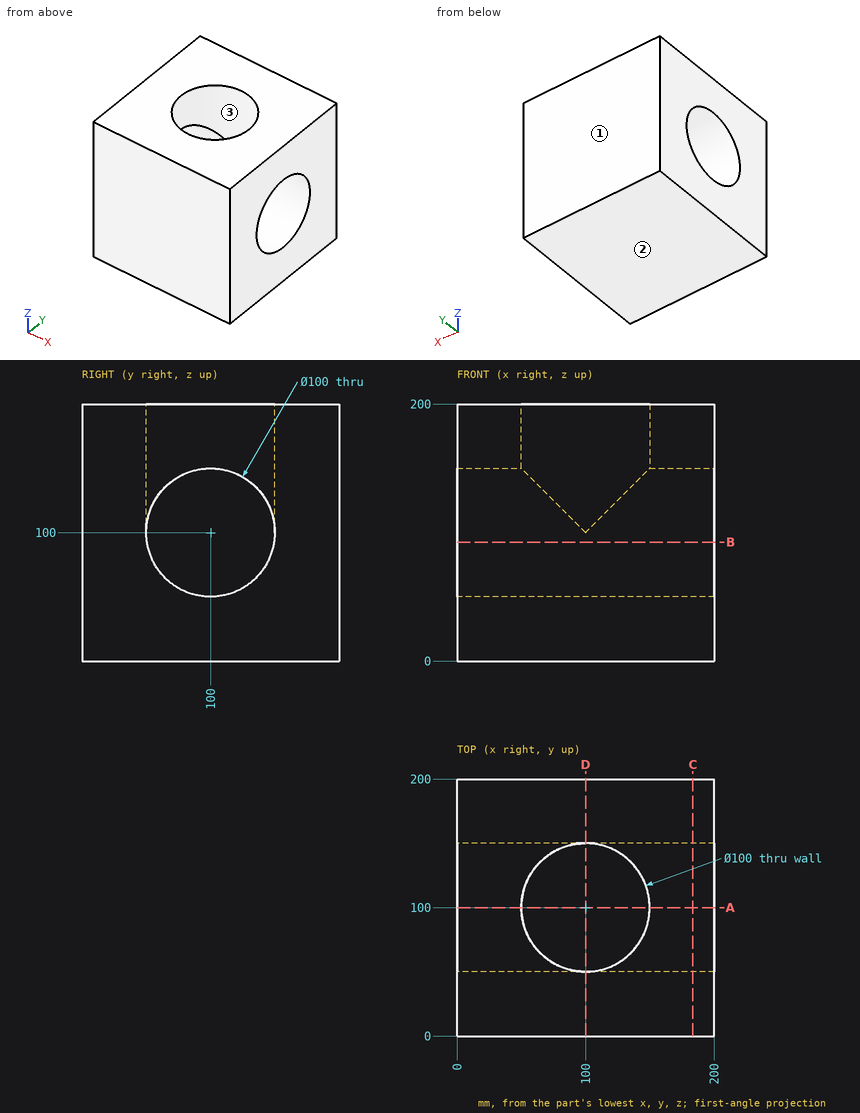
Can you work these out from the drawing? Everything is in mm from the part's minimum corner. Coordinates: 2 decimals unless noted, no trailing zeros. Loops run counter-clockwise (first coordinate to the right, second up) from the corner with the lowest first, then second, coordinate; pieces in that order, holes last.
1. Imagine slicing it at D-D, the plane x = 100. Please give me the cut outline in (y, z), and give its area (3 significant figures).
2. Imagine slicing it at C-C, the plane x = 183.5. Please give me the cut outline in (y, z), and give its area (3 significant figures).
3. Imagine slicing it at A-A, the plane y = 100. Please give me the cut outline in (x, z).
4. If we mould it in two halves opening along Y, with no side actions, what happens to the marked faces 1, 2 and 3? For each: pulls with the +Y half, pulls with the -Y half, needs draft (parallel to the pull), parting line crosses it, or undercut.
5. Imagine slicing it at B-B, the plane z = 92.5. Please give me the cut outline in (x, y), and give its area (3 significant figures).
6. I need wall thicknesses on L1, parallel to Y at x = 100, z = 148; L2, parallel to Y at x = 41, z = 56. Which ranges of each line are inside material? Lowest first, please.
Taken from the geometry:
1. outline: (0, 0) - (200, 0) - (200, 200) - (150, 200) - (150, 100) arc R50 cw to (50, 100) - (50, 200) - (0, 200) - close
1. area: 26,100 mm2
2. outline: (0, 0) - (200, 0) - (200, 200) - (0, 200) - close; hole circle Ø100 at (100, 100)
2. area: 32,100 mm2
3. outline: (0, 0) - (200, 0) - (200, 50) - (0, 50) - close; (0, 150) - (50, 150) - (50, 200) - (0, 200) - close; (150, 150) - (200, 150) - (200, 200) - (150, 200) - close
4. face 1: pulls with the +Y half
4. face 2: needs draft
4. face 3: undercut
5. outline: (0, 0) - (200, 0) - (200, 50.57) - (0, 50.57) - close; (0, 149.43) - (200, 149.43) - (200, 200) - (0, 200) - close
5. area: 20,200 mm2
6. L1: y = 0 to 50, 150 to 200
6. L2: y = 0 to 76.25, 123.75 to 200
